Design review of the part built by this model. Coordinates are the model's own, in mm. A direction names the side the tool comes from. Coordinates: 2 decimals unless noted, no trailing zeros. Write each loop counter-clockwise with the first axis right and the second up, starting at its lowest first coordinate (ties: lowest second). Pieces come first, ordered by that corner, then holes. Notation, with made-up numbers: (22, -24.75) -> (73, -24.75) arc R21 ccw to (73, -7.75) -> close; hole circle Ø1 at (47.5, 67). An arc over 180 degrees is marked (long way). Answer in a Markdown table with one row per item. Add a question column.
Item 1: For faces 4 (the face through (-8, 1, 5)), 5 (the face through (-1.096, 2.185, 1.726)), 6 (the face through (1, -6, 8)), list the 3-axis set-ups (+Z, -Z, +X, -X, +Y, -Y) from which the entire face can be reached by the end or side of a thin tool; tool diameter is ignored.
Item 2: Take a section at A-A, the plane y = -0.5. Write out the cut boundary in (x, z), and give its area (4 significant figures).
Item 3: Take a section at D-D, the plane z = 8. Write out the cut boundary in (x, y).
Item 4: Take a section at C-C, the plane z = 3.75. Write out the cut boundary in (x, y).
Item 5: To check wall thickness, follow line 1 (X direction, y = -0.5, z = 3.85); line 2 (X direction, y = -0.5, z = 2.05). State the ranges of each line that lie inside material, in increasing order.
Item 6: Clearance check with flat-ended pins moving along their axes: P1, Ø6.5, axis at y = 1.5, z = 9, coming from the +X side; P2, Ø2.5, axis at x = -0.5, y = -0.5, coming from the +Z side; P3, Ø1.6, axis at x = 0.5, y = 0.5, coming from the -Z side; P4, Ø1, axis at x = -0.5, z = 6, coming from the +Y side. State where each tip first meets the part, or that it passes through.
Item 7: Draft analysis for pull direction X (two halves, no side actions). For faces 1 (the face through (0.93, -0.05, 4.24)), 2 (the face through (-5, 6, 3)), 3 (the face through (-4, -5, 8)), state which applies: released by +X, released by -X, zero draft, split by the parting line, or undercut.
from build123d import *

# Parameters (mm, degrees)
F0_W     = 12
F0_H     = 12
F0_R     = 1.5
F0_H_2   = 2
F1_DEPTH = 5
F2_W     = 2
F2_H     = 12
F2_W_2   = 12
F2_H_2   = 2
F3_DEPTH = 6
F4_R     = 2.75
F5_DEPTH = 3.5
F6_SIZE  = 3
F7_SIZE  = 4
F8_R     = 5


with BuildPart() as f1:
    # F0 (on Top) → F1 (new body)
    with BuildSketch(Plane.XY):
        Rectangle(F0_W, F0_H)
        with Locations((-0.5, -0.5)):
            Circle(F0_R, mode=Mode.SUBTRACT)
        with Locations((0, -7)):
            Rectangle(F0_W, F0_H_2)
        Polygon((-6, -8), (-6, -6), (-6, 6), (-8, 6), (-8, -8), align=None)
    extrude(amount=F1_DEPTH)

    # F2 (on face) → F3 (join)
    with BuildSketch(Plane.XY.offset(5)):
        with Locations((-7, 0)):
            Rectangle(F2_W, F2_H)
        with Locations((0, -7)):
            Rectangle(F2_W_2, F2_H_2)
        with Locations((-7, -7)):
            Rectangle(F2_W, F2_H_2)
    extrude(amount=F3_DEPTH)

    # F4 (on face) → F5 (cut)
    with BuildSketch(Plane(origin=(0, 0, 0), x_dir=(1, 0, 0), z_dir=(0, 0, -1))):
        with Locations((-0.5, 0.5)):
            Circle(F4_R)
    extrude(amount=-F5_DEPTH, mode=Mode.SUBTRACT)

    # F6
    f6_edges = [f1.edges().sort_by_distance(p)[0] for p in [
        (-6, -6, 8),
    ]]
    chamfer(f6_edges, length=F6_SIZE)

    # F7
    f7_edges = [f1.edges().sort_by_distance(p)[0] for p in [
        (-8, -8, 5.5),
    ]]
    chamfer(f7_edges, length=F7_SIZE)

    # F8
    f8_edges = [f1.edges().sort_by_distance(p)[0] for p in [
        (6, 6, 2.5),
    ]]
    fillet(f8_edges, radius=F8_R)


solid = f1.part
Answers:
| question | item | result |
|---|---|---|
| 1 | face 4 | +Z, -Z, -X, +Y, -Y |
| 1 | face 5 | -Z |
| 1 | face 6 | +Z, +X, +Y |
| 2 | outline | (-8, 0) -> (-3.25, 0) -> (-3.25, 3.5) -> (-2, 3.5) -> (-2, 5) -> (-6, 5) -> (-6, 11) -> (-8, 11) -> close; (1, 3.5) -> (2.25, 3.5) -> (2.25, 0) -> (6, 0) -> (6, 5) -> (1, 5) -> close |
| 2 | area | 58.25 mm^2 |
| 3 | outline | (-8, -4) -> (-4, -8) -> (6, -8) -> (6, -6) -> (-3, -6) -> (-6, -3) -> (-6, 6) -> (-8, 6) -> close |
| 4 | outline | (-8, -4) -> (-4, -8) -> (6, -8) -> (6, 1) arc R5 ccw to (1, 6) -> (-8, 6) -> close; hole circle Ø3 at (-0.5, -0.5) |
| 5 | line 1 | x = -8 to -2, 1 to 6 |
| 5 | line 2 | x = -8 to -3.25, 2.25 to 6 |
| 6 | P1 | stops at x = -6 |
| 6 | P2 | passes through |
| 6 | P3 | stops at z = 3.5 |
| 6 | P4 | stops at y = -6 |
| 7 | face 1 | undercut |
| 7 | face 2 | zero draft |
| 7 | face 3 | released by +X |
